Here's the drawing with two shaded views (mm, measured from the low corner). I have some questions. A direction names the side the tool comes from. Give positions to 0.01 mm unless a question says otherwise; leave off trailing zeros. Write each loop counter-clockwise with the first axis right and the second up, starting at its lowest first coordinate (ties: lowest second). Pieces come first, ordered by that corner, then holes. Notation, with made-up numbers: M 52,14.5 L 74,14.5 A18 ccw 74,32.5 Z; hole C 81.5,7 d2. An arc over 180 degrees is marked long. Use one line per item in the form item = value. Start each with the question number.
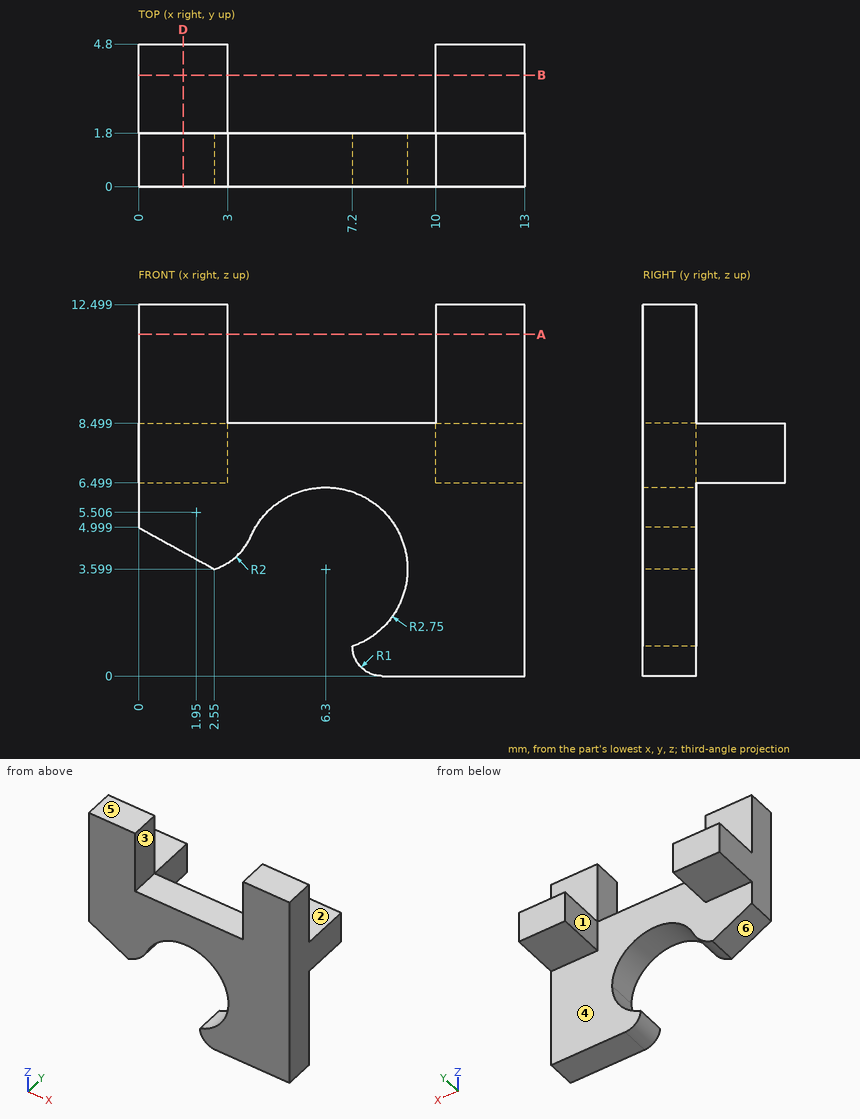
1) Suppose I cut it at B-B, the plane y = 3.75. List the corners of the cut face in (x, z) for me, and give its area (3 significant figures).
2) Thinking about a two-plate mould opening in X: for the marked faces 4, 5 and 6, which applies, released by +X, released by -X, zero draft, split by the parting line, or undercut?
3) Suppose I cut it at A-A, the plane z = 11.5. List the corners of the cut face in (x, y) for me.
4) Please list where these lines run through material, in increasing order: line 1 (X direction, y = 1.2, z = 9.25); line 2 (Z direction, x = 2.75, y = 2.45); line 3 (Z direction, x = 9.75, y = 0.4).
5) Suppose I cut it at D-D, the plane x = 1.5. List the corners of the cut face in (y, z) for me (1 decimal), and give its area (3 significant figures).
6) Will these pins go through, and if not, where does the flat tip stop? P1, Ø1.5, axis at x = 11.5, y = 3, coming from the -Z side; P2, Ø4, axis at x = 4.5, z = 4, coming from the +Y side; P3, Ø6, axis at x = 8.5, z = 11, coming from the +Y side; P4, Ø1.5, axis at x = 1.5, y = 3, coming from the +Z side.
7) On a 3-axis mill with a long thin cutter (end or side, diameter ignored), from which of +Z, -Z, +X, -X, +Y, -Y can I reach the whole of each face in a straight line? I mean the marked faces 1, 2 and 3. Say none if no direction works.
Checks:
q1.outline = M 0,6.5 L 3,6.5 L 3,8.5 L 0,8.5 Z; M 10,6.5 L 13,6.5 L 13,8.5 L 10,8.5 Z
q1.area = 12.0 mm^2
q2.face_4 = undercut
q2.face_5 = zero draft
q2.face_6 = released by -X
q3.outline = M 0,0 L 3,0 L 3,1.8 L 0,1.8 Z; M 10,0 L 13,0 L 13,1.8 L 10,1.8 Z
q4.line_1 = 0 to 3, 10 to 13
q4.line_2 = 6.5 to 8.5
q4.line_3 = 0 to 8.5
q5.outline = M 0,4.2 L 1.8,4.2 L 1.8,6.5 L 4.8,6.5 L 4.8,8.5 L 1.8,8.5 L 1.8,12.5 L 0,12.5 Z
q5.area = 21.0 mm^2
q6.P1 = 6.5
q6.P2 = 1.8
q6.P3 = 4.8
q6.P4 = 8.5
q7.face_1 = +Z, -Z, +Y
q7.face_2 = +Z, +X, -X, +Y
q7.face_3 = +Z, +Y, -Y
